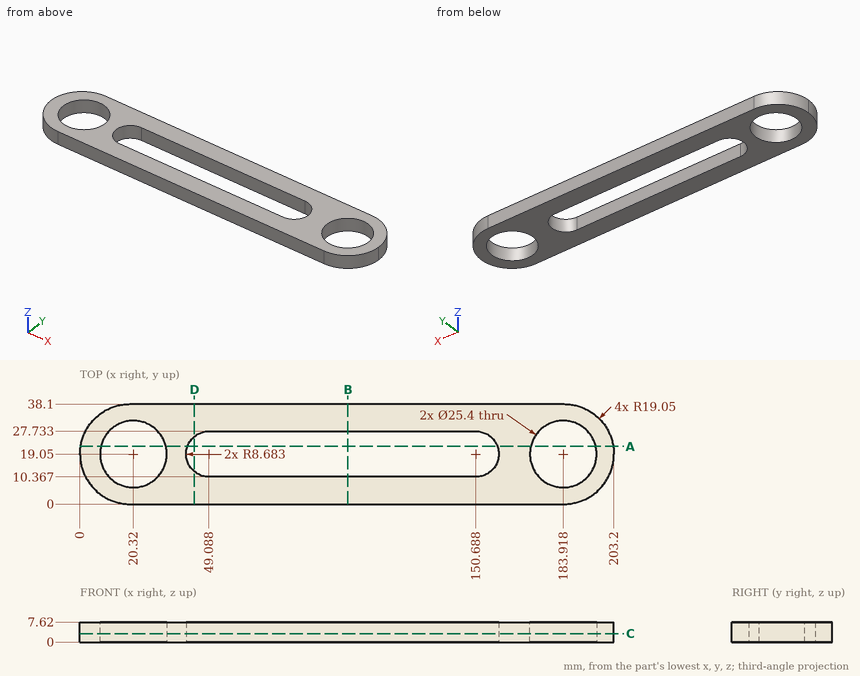
Source: three-view drawing plus pictorial views. Frame: mm from the lowest corner of the part. Round coordinates to 2 decimals unless told otherwise and drop trailing zeros. Loops run counter-clockwise (first coordinate to the right, second up) from the corner with the lowest first, then second, coordinate; pieces in that order, holes last. Notation, with made-up numbers: M -39.5,33.25 L 4.5,33.25 A26 ccw 4.5,51.25 Z; hole C 72,-2 d8. An arc over 180 degrees is marked long. Answer as CSV lines item,"result". Start each with the question number.
(1) Section B-B, the plane x = 102. Output: boundary loops of the cut face in (y, z).
(2) Line query: line 1 (Y direction, x = 93, z = 4.75); line 2 (Y direction, x = 20.32, z = 4.75); line 3 (X direction, y = 18, z = 4.5) (1 decimal). Output: solid intervals per line, ascending. Write a range as [from, to].
(3) Section D-D, the plane x = 43.5. Output: boundary loops of the cut face in (y, z) (1 decimal).
(4) Section C-C, the plane z = 3.25. State how many separate pieces and enclosed holes the cut face has, plus the area to 3 significant figures.
(5) Section A-A, the plane y = 22. Output: boundary loops of the cut face in (x, z) (1 decimal).
(6) First-contact query: pin 1 (1 mm diameter, centred on y = 8, z = 6.5, fed in from -X). Flat tip, straight axial feed; report the tip coordinate or a pass-through.
Values found:
1,outline,"M 0,0 L 10.37,0 L 10.37,7.62 L 0,7.62 Z; M 27.73,0 L 38.1,0 L 38.1,7.62 L 27.73,7.62 Z"
2,line 1,"y = [0, 10.37], [27.73, 38.1]"
2,line 2,"y = [0, 6.35], [31.75, 38.1]"
2,line 3,"x = [0, 7.7], [33, 40.5], [159.3, 171.3], [196.6, 203.2]"
3,outline,"M 0,0 L 12.4,0 L 12.4,7.6 L 0,7.6 Z; M 25.7,0 L 38.1,0 L 38.1,7.6 L 25.7,7.6 Z"
4,separate pieces,"1"
4,enclosed holes,"3"
4,area,"4,420 mm²"
5,outline,"M 0.2,0 L 8,0 L 8,7.6 L 0.2,7.6 Z; M 32.7,0 L 40.9,0 L 40.9,7.6 L 32.7,7.6 Z; M 158.9,0 L 171.6,0 L 171.6,7.6 L 158.9,7.6 Z; M 196.3,0 L 203,0 L 203,7.6 L 196.3,7.6 Z"
6,pin 1,"stops at x = 3.19"
